from build123d import *
from build123d.topology import SkipClean

# Parameters (mm, degrees)
SKETCH_2_R               = 24
SKETCH_2_R_2             = 15.5
SKETCH_2_R_3             = 1
EXTRUDE_1_DEPTH          = 1.5
EXTRUDE_START            = 12
SKETCH_4_R               = 17
SKETCH_4_R_2             = 15.5
EXTRUDE_3_DEPTH          = 12
EXTRUDE_START_2          = -1.2
SKETCH_5_R               = 17
SKETCH_5_R_2             = 5
EXTRUDE_4_DEPTH          = 1.5
SKETCH_6_W               = 23
SKETCH_6_H               = 48
CUT_EXTRUDE_1_DEPTH      = 8
SKETCH_7_R               = 6.5
SKETCH_7_R_2             = 5
EXTRUDE_5_DEPTH          = 8
CUT_EXTRUDE_2_DEPTH      = 10
CUT_EXTRUDE_2_DEPTH_BACK = 10
SKETCH_8_R               = 1.5


with BuildPart() as part:
    # Sketch 2 → Extrude 1 (new body)
    with BuildSketch(Plane(origin=(0, 0, 0), x_dir=(1, 0, 0), z_dir=(0, 1, 0))):
        with Locations(Location((0, 0, 0), (0, 0, 270))):
            Circle(SKETCH_2_R)
        with Locations(Location((0, 0, 0), (0, 0, 270))):
            Circle(SKETCH_2_R_2, mode=Mode.SUBTRACT)
        with Locations(Location((-15, 15, 0), (0, 0, 270))):
            Circle(SKETCH_2_R_3, mode=Mode.SUBTRACT)
        with Locations(Location((15, 15, 0), (0, 0, 270))):
            Circle(SKETCH_2_R_3, mode=Mode.SUBTRACT)
        with Locations(Location((-15, -15, 0), (0, 0, 270))):
            Circle(SKETCH_2_R_3, mode=Mode.SUBTRACT)
        with Locations(Location((15, -15, 0), (0, 0, 270))):
            Circle(SKETCH_2_R_3, mode=Mode.SUBTRACT)
    extrude(amount=EXTRUDE_1_DEPTH)

    # Sketch 4 → Extrude 3 (add)
    with SkipClean():  # the faces are left unmerged after this step: merging them gives an invalid solid
        with BuildSketch(Plane.XZ.offset(EXTRUDE_START)):
            with Locations(Location((0, 0, 0), (0, 0, 90))):
                Circle(SKETCH_4_R)
            with Locations(Location((0, 0, 0), (0, 0, 270))):
                Circle(SKETCH_4_R_2, mode=Mode.SUBTRACT)
        extrude(amount=-EXTRUDE_3_DEPTH)

    # Sketch 5 → Extrude 4 (add)
    with SkipClean():  # the faces are left unmerged after this step: merging them gives an invalid solid
        with BuildSketch(Plane.XZ.offset(12).offset(EXTRUDE_START_2)):
            with Locations(Location((0, 0, 0), (0, 0, 90))):
                Circle(SKETCH_5_R)
            with Locations(Location((0, 0, 0), (0, 0, 270))):
                Circle(SKETCH_5_R_2, mode=Mode.SUBTRACT)
        extrude(amount=-EXTRUDE_4_DEPTH)

    # Sketch 6 → Cut-Extrude 1 (cut)
    with SkipClean():  # the faces are left unmerged after this step: merging them gives an invalid solid
        with BuildSketch(Plane(origin=(0, 1.5, 0), x_dir=(1, 0, 0), z_dir=(0, 1, 0))):
            Rectangle(SKETCH_6_W, SKETCH_6_H)
        extrude(amount=-CUT_EXTRUDE_1_DEPTH, mode=Mode.SUBTRACT)
    add(part.part.scale(1), mode=Mode.REPLACE)  # the faces are merged on a copy

    # Sketch 7 → Extrude 5 (add)
    with BuildSketch(Plane(origin=(0, -9.3, 0), x_dir=(1, 0, 0), z_dir=(0, 1, 0))):
        with Locations(Location((0, 0, 0), (0, 0, 90))):
            Circle(SKETCH_7_R)
        with Locations(Location((0, 0, 0), (0, 0, 90))):
            Circle(SKETCH_7_R_2, mode=Mode.SUBTRACT)
    extrude(amount=EXTRUDE_5_DEPTH)

    # Sketch 8 → Cut-Extrude 2 (cut, two sides: drawn at the far end of the back side and taken through both)
    with BuildSketch(Plane.XY.offset(-CUT_EXTRUDE_2_DEPTH_BACK)):
        with Locations(Location((0, -4.3, 0), (0, 0, 180))):
            Circle(SKETCH_8_R)
    extrude(amount=CUT_EXTRUDE_2_DEPTH + CUT_EXTRUDE_2_DEPTH_BACK, mode=Mode.SUBTRACT)


solid = part.part
Can you work these out from the model? Positions are in its coordinate system, mm. A direction names the side the tool comes from. Round coordinates to 2 decimals unless told otherwise and drop trailing zeros. Order: outer loops, then holes, each group sorted by start corner. A loop starts at its lowest first (then second) coordinate and runs counter-clockwise, first axis right, second up. Notation, with made-up numbers: (78, 14) -> (112, 14) arc R31 ccw to (112, 44) -> close; hole circle Ø11 at (60, 53). An arc over 180 degrees is marked (long way). Write each question's results on one line, items separated by ' | '. Start each with the question number.
Item 1: Please list where these lines run through material, in increasing order: L1, parallel to X at y = 0.6, z = -15 (3 decimals); L2, parallel to X at y = -10, z = 0; L3, parallel to X at y = -8, z = -1.
Item 2: If we section it at B-B, the plane y = -8.5: Write out the boundary of the cut face in (x, z), then the cut area to 3 significant figures.
Item 3: If we section it at C-C, the plane z = -3.5: Write out the boundary of the cut face in (x, y).
Item 4: Thinking about a two-plate mould opening in X: for faces 4 (the cylindrical face through (-24, 1, 0)), 5 (the cylindrical face through (15.368, -11.408, 2.018)), 6 (the flat face through (11.5, 0.2, 13.4)), 7 (the flat face through (18, 1.5, 0)), which applies, +X half, -X half, draft (parallel to the pull), parting line (faces both ways), or undercut?
Item 5: Will these pins go through, and if not, where does the flat tip stop? pin 1 (1.5 mm diameter, centred on x = -14.5, y = -7, fed in from -Z); pin 2 (2.5 mm diameter, centred on y = -3, z = 16, fed in from +X); pin 3 (18.5 mm diameter, centred on x = 0, z = 0, fed in from -Y); pin 4 (6 mm diameter, centred on y = -10, z = -16.5, fed in from +X).
Item 6: Which directions (+Z, -Z, +X, -X, +Y, -Y) give clear straight access to the entire face, cutting with the end or side of a thin tool? Please do faces 1 (the flat face through (-18, 0, 0)), 2 (the cylindrical face through (-1.95, -5.36, -6.2)), 3 (the flat face through (5, -1.3, -2)).
Item 7: If we section it at A-A, the plane x = 0: Write out the boundary of the cut face in (y, z), then the cut area to 3 significant figures.
Item 8: If we section it at D-D, the plane y = -4.3: Write out the boundary of the cut face in (x, z).
Results:
1) L1: x = -18.735 to -16, -14 to -11.5, 11.5 to 14, 16 to 18.735 | L2: x = -17 to -5, 5 to 17 | L3: x = -16.97 to -15.47, -6.42 to -4.9, 4.9 to 6.42, 15.47 to 16.97
2) outline: circle Ø34 at (0, 0); circle Ø13 at (0, 0); hole circle Ø31 at (0, 0); hole circle Ø10 at (0, 0) | area: 207 mm2
3) outline: (-23.74, 0) -> (-16.64, 0) -> (-16.64, -12) -> (-15.1, -12) -> (-15.1, -10.8) -> (-3.57, -10.8) -> (-3.57, -1.3) -> (-5.48, -1.3) -> (-5.48, -9.3) -> (-15.1, -9.3) -> (-15.1, 1.5) -> (-23.74, 1.5) -> close; (3.57, -10.8) -> (15.1, -10.8) -> (15.1, -12) -> (16.64, -12) -> (16.64, 0) -> (23.74, 0) -> (23.74, 1.5) -> (15.1, 1.5) -> (15.1, -9.3) -> (5.48, -9.3) -> (5.48, -1.3) -> (3.57, -1.3) -> close
4) face 4: -X half | face 5: undercut | face 6: undercut | face 7: draft
5) pin 1: stops at z = -10 | pin 2: passes through | pin 3: stops at y = -10.8 | pin 4: stops at x = 10.33
6) face 1: -X, -Y | face 2: +Y | face 3: +Z, -Z, +Y
7) outline: (-12, -17) -> (-6.5, -17) -> (-6.5, -15.5) -> (-9.3, -15.5) -> (-9.3, -6.5) -> (-5.8, -6.5) -> (-5.8, -5) -> (-10.8, -5) -> (-10.8, -15.5) -> (-12, -15.5) -> close; (-12, 15.5) -> (-10.8, 15.5) -> (-10.8, 5) -> (-5.8, 5) -> (-5.8, 6.5) -> (-9.3, 6.5) -> (-9.3, 15.5) -> (-6.5, 15.5) -> (-6.5, 17) -> (-12, 17) -> close; (-2.8, -6.5) -> (-1.3, -6.5) -> (-1.3, -5) -> (-2.8, -5) -> close; (-2.8, 5) -> (-1.3, 5) -> (-1.3, 6.5) -> (-2.8, 6.5) -> close | area: 63.0 mm2
8) outline: (-11.5, -12.52) -> (-11.5, -10.39) arc R15.5 cw to (-11.5, 10.39) -> (-11.5, 12.52) arc R17 ccw to start; (-1.5, -6.32) -> (-1.5, -4.77) arc R5 cw to (-1.5, 4.77) -> (-1.5, 6.32) arc R6.5 ccw to start; (1.5, -6.32) arc R6.5 ccw to (1.5, 6.32) -> (1.5, 4.77) arc R5 cw to (1.5, -4.77) -> close; (11.5, -12.52) arc R17 ccw to (11.5, 12.52) -> (11.5, 10.39) arc R15.5 cw to (11.5, -10.39) -> close
